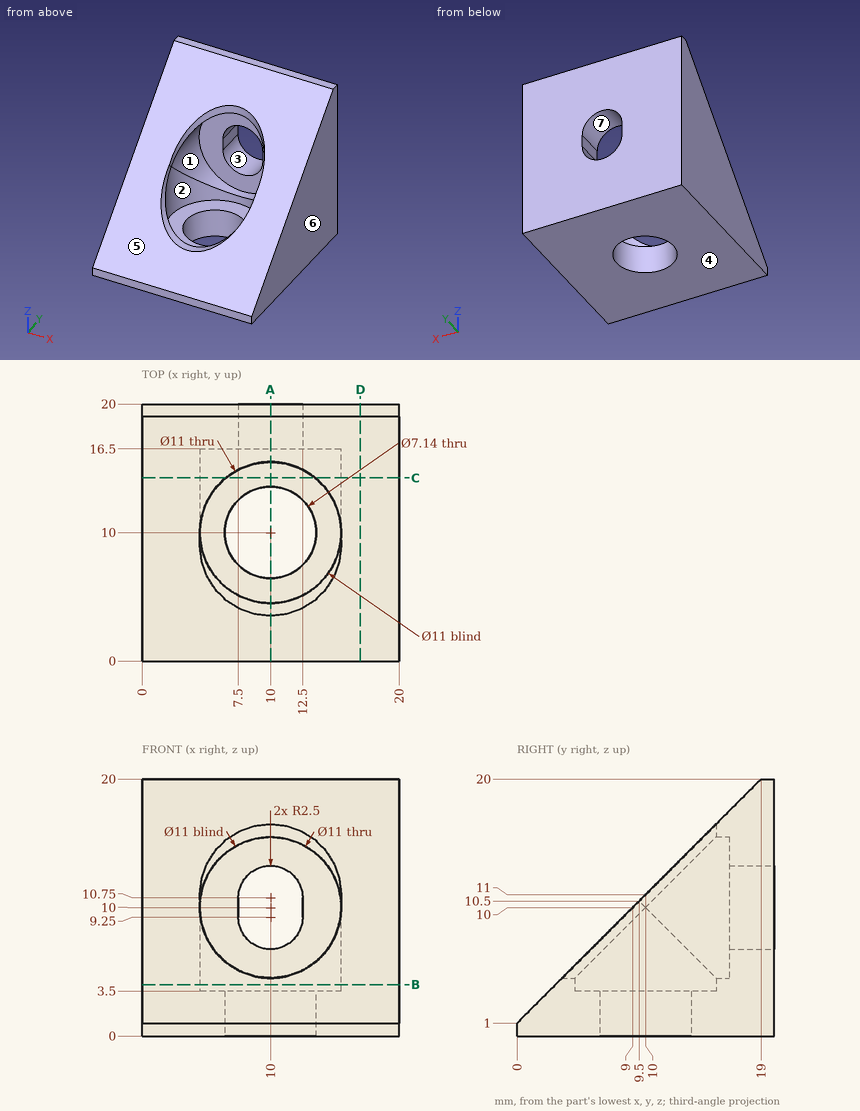
Job drawing, mm, ordinate dimensions from the low corner. One solid piece. A direction names the side the tool comes from. Round coordinates to 2 decimals unless told otherwise and drop trailing zeros. Loops run counter-clockwise (first coordinate to the right, second up) from the corner with the lowest first, then second, coordinate; pieces in that order, holes last.
(1) Cut at A-A (x = 10). Give the cut face in (y, z), plus the area to 3 significant figures.
(2) Cut at D-D (x = 17). Give the cut face in (y, z).
(3) Drop flat-ended pins along their axis: pin 1 (10 mm diameter, centred on x = 10, y = 10, fed in from +Z); pin 2 (3.5 mm diameter, centred on x = 7.5, z = 12, fed in from -Y); pin 3 (3 mm diameter, centred on x = 8.5, y = 14.5, fed in from +Z). Give the stop position or say it passes through.
(4) Which spindle directions (+Z, -Z, +X, -X, +Y, -Y) get a long thin tool onto all of the face, cutting with end or side? Do the marked faces 1, 2 and 3. Say none if no direction does.
(5) Two-plate mould, pull along Z, no slides. Class the marked faces 4, 5, 6 and 7: +Z half, -Z half, draft (parallel to the pull), parting line (faces both ways), or undercut.
(6) Cut at C-C (y = 14.25). Give the cut face in (x, z), plus the area to 3 significant figures.
(7) Cut at B-B (z = 4). Give the cut face in (x, y).
(8) Wall check: line 1 along X through (y, z) = (13.75, 10); line 2 along X through (y, z) = (7.25, 2.25); line 3 along Y through (x, z) = (14.25, 12.25). Give the ranges that are in metal, low to high.
Findings below:
1. outline: (0, 0) - (6.43, 0) - (6.43, 3.5) - (4.5, 3.5) - (4.5, 4.5) - (3.5, 4.5) - (0, 1) - close; (13.57, 0) - (20, 0) - (20, 6.75) - (16.5, 6.75) - (16.5, 4.5) - (15.5, 4.5) - (15.5, 3.5) - (13.57, 3.5) - close; (15.5, 15.5) - (16.5, 15.5) - (16.5, 13.25) - (20, 13.25) - (20, 20) - (19, 20) - (15.5, 16.5) - close
1. area: 77.8 mm2
2. outline: (0, 0) - (20, 0) - (20, 20) - (19, 20) - (0, 1) - close
3. pin 1: stops at z = 3.5
3. pin 2: stops at y = 16.5
3. pin 3: stops at z = 17
4. face 1: -Y
4. face 2: +Z
4. face 3: +Y, -Y
5. face 4: -Z half
5. face 5: +Z half
5. face 6: draft
5. face 7: undercut
6. outline: (0, 0) - (20, 0) - (20, 15.25) - (13.49, 15.25) - (13.49, 14.25) arc R5.5 cw to (13.49, 5.75) - (13.49, 3.5) - (6.51, 3.5) - (6.51, 5.75) arc R5.5 cw to (6.51, 14.25) - (6.51, 15.25) - (0, 15.25) - close
6. area: 199 mm2
7. outline: (0, 3) - (20, 3) - (20, 20) - (0, 20) - close; hole circle Ø11 at (10, 10)
8. line 1: x = 0 to 4.5, 15.5 to 20
8. line 2: x = 0 to 7.72, 12.28 to 20
8. line 3: y = 16.5 to 20
